Autodesk Inventor part; units mm, degrees
ref_plane "YZ Plane" through (0, 0, 0) normal (1, 0, 0) x (0, 1, 0)
ref_plane "XZ Plane" through (0, 0, 0) normal (0, 1, 0) x (-1, 0, 0)
ref_plane "XY Plane" through (0, 0, 0) normal (0, 0, 1) x (1, 0, 0)
sketch "Sketch1" plane through (0, 0, 0) normal (1, 0, 0) x (0, 1, 0)
  line L0 (0, 0) -> (50.8, 0) construction
  line L1 (50.8, 0) -> (50.8, -50.8) construction
  line L2 (50.8, -50.8) -> (0, -50.8) construction
  line L3 (0, -50.8) -> (0, 0) construction
  line L4 (0, 0) -> (50.8, 0)
  line L5 (50.8, 0) -> (50.8, -9.525)
  line L6 (0, 0) -> (0, -50.8)
  line L7 (50.8, -25.4) -> (50.8, -38.1)
  line L8 (50.8, -38.1) -> (25.4, -50.8)
  line L9 (25.4, -50.8) -> (0, -50.8)
  circle A0 centre (38.1, -15.875) radius 3.175 construction
  line L10 (50.8, -9.525) -> (37.351, -12.7896)
  line L11 (50.8, -25.4) -> (36.7415, -18.7447)
  arc A1 (37.351, -12.7896) -> (36.7415, -18.7447) centre (38.1, -15.875) ccw
  dimension "d0" = 50.8
  dimension "d1" = 50.8
  dimension "d2" = 9.525
  dimension "d3" = 12.7
  dimension "d6" = 6.35
  dimension "d7" = 12.7
  dimension "d8" = 15.875
  dimension "d22" = 25.4
  dimension "d23" = 12.7
extrude "Extrusion1" add sketch "Sketch1" along normal blind 3.175
sketch "Sketch2" plane through (3.175, 0, 0) normal (1, 0, 0) x (0, 0, -1)
  line L0 (0, 50.8) -> (0, 0)
  line L1 (0, 0) -> (50.8, 0)
  point P0 (12.7, 12.7)
  point P1 (38.1, 12.7)
  dimension "d11" = 12.7
  dimension "d12" = 12.7
  dimension "d13" = 12.7
  dimension "d14" = 38.1
hole "Hole1" at (3.175, 12.7, -12.7) at (3.175, 12.7, -38.1) direction (-1, 0, 0) diameter 6.35 end through all
properties part number "pickup arm tab with hook" material "Aluminum 6061"
The model under review builds one solid part; all positions refer to its coordinate system, in mm. A direction names the side the tool comes from. Give positions to 0.01 mm unless a question says otherwise; leave off trailing zeros. Order: outer loops, then holes, each group sorted by start corner. A loop starts at its lowest first (then second) coordinate and runs counter-clockwise, first axis right, second up. Notation, with made-up numbers: M -2,17 L 16,17 A15 ccw 16,38 Z; hole C 89.25,25 d5. An arc over 180 degrees is marked long. Answer in a Markdown table with one row per item. Add a question column.
1. Add section B-B on y = 12.7. State the section outline as (x, z) points (3 decimals), plus the area to 3 significant figures.
2. Add section A-A on x = 2.5. Count the separate pieces of the cut face and the enclosed holes in it, plus the area to 3 significant figures.
3. Add section D-D on z = -45. State the section outline as (x, y) points (3 decimals).
4. Machinability: for faces 4 (the flat face through (2, 0, -25)), 5 (the flat face through (1.565, 44.17, -11.134)), which of the approach directions +Z, -Z, +X, -X, +Y, -Y give a long, thin tool a straight path to every point of the face, cutting with its end or side? Answer none if there is none.
5. For pin 1 Ø8 at (y, z) = (32.5, -38) entering from -X, flat-tipped, find the tip position at first contact; note if it passes through.
6. To check wall thickness, follow line 1 along Z through (x, y) = (1.95, 12.7) (3 decimals); line 2 along Z through (x, y) = (0.2, 48.5); line 3 along Z through (x, y) = (1.25, 38). State the ranges of each line that lie inside material, in increasing order.
7. Add section C-C on y = 31. State the section outline as (x, z) points (3 decimals).
8. Mouldability with a two-part tool opening along Z and no side actions: class faces 1 (the flat face through (2, 25, 0)), 2 (the flat face through (3.175, 25, -25)), 3 (the cylindrical face through (1.565, 34.936, -15.606)) as released by +Z, released by -Z, zero draft, split by the parting line, or undercut.
The answers:
| question | item | result |
|---|---|---|
| 1 | outline | M 0,-50.8 L 3.175,-50.8 L 3.175,-41.275 L 0,-41.275 Z; M 0,-34.925 L 3.175,-34.925 L 3.175,-15.875 L 0,-15.875 Z; M 0,-9.525 L 3.175,-9.525 L 3.175,0 L 0,0 Z |
| 1 | area | 121 mm2 |
| 2 | separate pieces | 1 |
| 2 | enclosed holes | 2 |
| 2 | area | 2,200 mm2 |
| 3 | outline | M 0,0 L 3.175,0 L 3.175,37 L 0,37 Z |
| 4 | face 4 | +Z, -Z, +X, -X, -Y |
| 4 | face 5 | +X, -X, +Y |
| 5 | pin 1 | x = 0 |
| 6 | line 1 | -50.8 to -41.275, -34.925 to -15.875, -9.525 to 0 |
| 6 | line 2 | -39.25 to -24.31, -10.08 to 0 |
| 6 | line 3 | -44.5 to -19.34, -12.63 to 0 |
| 7 | outline | M 0,-48 L 3.175,-48 L 3.175,0 L 0,0 Z |
| 8 | face 1 | released by +Z |
| 8 | face 2 | zero draft |
| 8 | face 3 | undercut |
